Autodesk Fusion 360 part; units mm, degrees
sketch "Sketch1" plane through (0, 0, 0) normal (0, 0, 1) x (1, 0, 0)
  line L0 (0, 0) -> (20, 0)
  line L1 (20, 25) -> (2, 25)
  line L2 (0, 23) -> (0, 0)
  line L3 (0, 25) -> (32.3455, 25)
  line L4 (34.03, 21.9219) -> (20, 0)
  arc A0 (2, 25) -> (0, 23) centre (2, 23) ccw
  arc A1 (34.03, 21.9219) -> (32.3455, 25) centre (32.3455, 23) ccw
  line L5 (20, 25) -> (20, 0) construction
  line L6 (10, 0) -> (10, 25) construction
  line L7 (7.997, 0) -> (11.997, 0)
  line L8 (11.997, 0) -> (11.997, -5)
  line L9 (11.997, -5) -> (7.997, -5)
  line L10 (7.997, -5) -> (7.997, 0)
  line L11 (12.6, 20.6) -> (7.4, 20.6)
  line L12 (7.4, 20.6) -> (7.4, 23.1)
  line L13 (7.4, 23.1) -> (12.6, 23.1)
  line L14 (12.6, 23.1) -> (12.6, 20.6)
  line L15 (12.6, 20.6) -> (7.4, 23.1) construction
  line L16 (7.4, 20.6) -> (12.6, 23.1) construction
  line L17 (12.6, 3.5) -> (7.4, 3.5)
  line L18 (7.4, 3.5) -> (7.4, 1.2)
  line L19 (7.4, 1.2) -> (12.6, 1.2)
  line L20 (12.6, 1.2) -> (12.6, 3.5)
  line L21 (12.6, 3.5) -> (7.4, 1.2) construction
  line L22 (7.4, 3.5) -> (12.6, 1.2) construction
  line L23 (18.4, 1.2) -> (15.3, 1.2)
  line L24 (15.3, 1.2) -> (15.3, 3.5)
  line L25 (15.3, 3.5) -> (18.4, 3.5)
  line L26 (18.4, 3.5) -> (18.4, 1.2)
  line L27 (1.6, 3.5) -> (1.6, 1.2)
  line L28 (1.6, 1.2) -> (4.7, 1.2)
  line L29 (4.7, 1.2) -> (4.7, 3.5)
  line L30 (4.7, 3.5) -> (1.6, 3.5)
  point P0 (36, 25)
  point P1 (10, 21.85)
  point P2 (10, 2.35)
  dimension "d1" = 20
  dimension "d2" = 25
  dimension "d3" = 36
  dimension "d4" = 2
  dimension "d5" = 2
  dimension "d6" = 4
  dimension "d7" = 5
  dimension "d8" = 5.2
  dimension "d9" = 2.5
  dimension "d10" = 1.9
  dimension "d11" = 5.2
  dimension "d12" = 2.3
  dimension "d13" = 1.2
  dimension "d16" = 3.1
  dimension "d17" = 2.3
  dimension "d18" = 1.6
extrude "Extrude1" add sketch "Sketch1" along normal blind 1.5 contours L0 L1 L2 L3 L4 A0 A1 L7 makes body 1
extrude "Extrude2" add sketch "Sketch1" along normal blind 1.4 separate body makes body 2
extrude "Extrude3" cut sketch "Sketch1" along normal blind 0.5 contours L0 L7 L8 L9 L10 bodies 2
delete_body "RemoveBody1" bodies 1
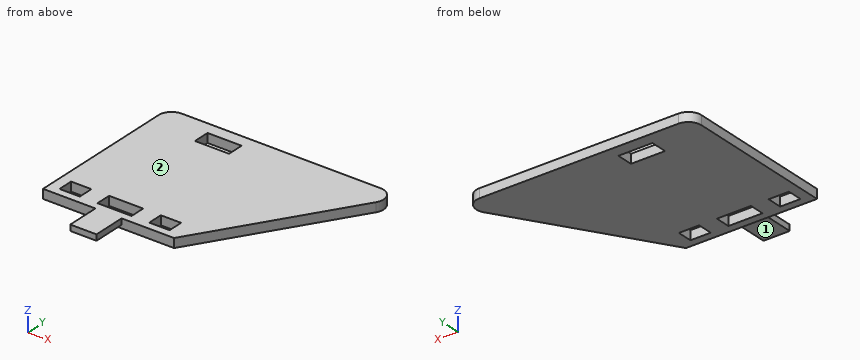
The model under review builds one solid part; all positions refer to its coordinate system, in mm. Face numbers are marked on the shaded views. A direction names the side the tool comes from. Give positions to 0.01 mm unless a question says otherwise; leave off trailing zeros. Write each loop counter-clockwise with the first axis right and the second up, starting at its lowest first coordinate (ties: lowest second). Pieces come first, ordered by that corner, then holes. Notation, with made-up numbers: M -6,-12 L 41,-12 A27 ccw 41,17 Z; hole C 47,-19 d6. An arc over 180 degrees is marked long. Write item = value, one per line. Start each with the question number.
Q1. We need section B-B (x = 11.5). State the section outline as (y, z) points, plus the area to 3 significant figures.
Q2. Clearance check with flat-ended pins moving along their axes: pin 1 (3 mm diameter, centred on x = 10.5, y = -2.5, fed in from -Z); pin 2 (0.7 mm diameter, centred on y = -3.5, z = 1, fed in from -X). State where each tip first meets the part, or that it passes through.
Q3. We need section A-A (z = 0.85). State the section outline as (x, y) points.
Q4. We need section C-C (y = 0.5). State the section outline as (x, z) points, plus the area to 3 significant figures.
Q5. Machinability: for the marked faces 1 and 2, which of the approach directions +Z, -Z, +X, -X, +Y, -Y give a long, thin tool a straight path to every point of the face, cutting with its end or side? Answer none if there is none.
Q6. We need section D-D (x = 30). State the section outline as (y, z) points, plus the area to 3 significant figures.
Q7. For line 1 (Y direction, x = 11, z = 0.2); line 2 (Y direction, x = 10, z = 1.3); line 3 (X direction, y = 3, z = 1.35), list the stretches that pass through material, from the lowest coordinate up.
Result set:
q1.outline = M -5,0.5 L 0,0.5 L 0,0 L 1.2,0 L 1.2,1.4 L -5,1.4 Z; M 3.5,0 L 20.6,0 L 20.6,1.4 L 3.5,1.4 Z; M 23.1,0 L 25,0 L 25,1.4 L 23.1,1.4 Z
q1.area = 32.8 mm2
q2.pin_1 = 0.5
q2.pin_2 = 8
q3.outline = M 0,0 L 8,0 L 8,-5 L 12,-5 L 12,0 L 20,0 L 34.03,21.92 A2 ccw 32.35,25 L 2,25 A2 ccw 0,23 Z; hole M 1.6,1.2 L 4.7,1.2 L 4.7,3.5 L 1.6,3.5 Z; hole M 7.4,1.2 L 12.6,1.2 L 12.6,3.5 L 7.4,3.5 Z; hole M 7.4,20.6 L 12.6,20.6 L 12.6,23.1 L 7.4,23.1 Z; hole M 15.3,1.2 L 18.4,1.2 L 18.4,3.5 L 15.3,3.5 Z
q4.outline = M 0,0 L 20.32,0 L 20.32,1.4 L 0,1.4 Z
q4.area = 28.4 mm2
q5.face_1 = -Z, +X, -X, -Y
q5.face_2 = +Z, +X, -X, +Y, -Y
q6.outline = M 15.63,0 L 25,0 L 25,1.4 L 15.63,1.4 Z
q6.area = 13.1 mm2
q7.line_1 = 0 to 1.2, 3.5 to 20.6, 23.1 to 25
q7.line_2 = -5 to 1.2, 3.5 to 20.6, 23.1 to 25
q7.line_3 = 0 to 1.6, 4.7 to 7.4, 12.6 to 15.3, 18.4 to 21.92
